from build123d import *

# Parameters (mm, degrees)
SKETCH1_W               = 120
SKETCH1_H               = 100
BOSS_EXTRUDE1_DEPTH     = 5
SKETCH2_R               = 2.5
CUT_EXTRUDE1_DEPTH      = 6
CUT_EXTRUDE3_DEPTH      = 10
BOSS_EXTRUDE3_DEPTH     = 60
SKETCH8_W               = 20
SKETCH8_H               = 5
BOSS_EXTRUDE4_DEPTH     = 65
SKETCH9_R               = 2.5
CUT_EXTRUDE4_DEPTH      = 71
BOSS_EXTRUDE5_DEPTH     = 5
SKETCH11_W              = 5
SKETCH11_H              = 70
CUT_EXTRUDE6_DEPTH      = 1
CUT_EXTRUDE6_DEPTH_BACK = 120.643960247
SKETCH12_R              = 1.5
CUT_EXTRUDE7_DEPTH      = 66
CUT_EXTRUDE7_DEPTH_BACK = 6
SKETCH13_W              = 69.121998964
SKETCH13_H              = 5
BOSS_EXTRUDE6_DEPTH     = 10
SKETCH14_R              = 1.5
CUT_EXTRUDE8_DEPTH      = 61
SKETCH15_W              = 5
SKETCH15_H              = 15
BOSS_EXTRUDE7_DEPTH     = 10
SKETCH17_R              = 1.5
CUT_EXTRUDE9_DEPTH      = 61


with BuildPart() as part:
    # Sketch1 → Boss-Extrude1 (new body)
    with BuildSketch(Plane.XY):
        with Locations((60, 50)):
            Rectangle(SKETCH1_W, SKETCH1_H)
    extrude(amount=BOSS_EXTRUDE1_DEPTH)

    # Sketch2 → Cut-Extrude1 (cut, through all)
    with BuildSketch(Plane.XY.offset(5)):
        with Locations((50.878001036, 56.909722104)):
            Circle(SKETCH2_R)
        with BuildLine():
            ThreePointArc((85.579375435, 7.351023424), (95.403755905, 15.949898455), (103.154556632, 26.456286582))
            ThreePointArc((103.154556632, 26.456286582), (98.465291161, 44.232978888), (80.688598855, 39.543713418))
            ThreePointArc((80.688598855, 39.543713418), (76.268720755, 33.552467296), (70.66638809, 28.648976576))
            ThreePointArc((70.66638809, 28.648976576), (67.473905187, 10.543506327), (85.579375435, 7.351023424))
        make_face()
    extrude(amount=-CUT_EXTRUDE1_DEPTH, mode=Mode.SUBTRACT)

    # Sketch5 → Cut-Extrude3 (cut)
    with BuildSketch(Plane.XY.offset(5)):
        with BuildLine():
            Line((120, 70), (50.878001036, 70))
            ThreePointArc((50.878001036, 70), (43.464411706, 67.698330385), (38.657892056, 61.602728806))
            Line((38.657892056, 61.602728806), (15, 0))
            Line((15, 0), (0, 0))
            Line((0, 0), (0, 100))
            Line((0, 100), (120, 100))
            Line((120, 100), (120, 70))
        make_face()
    extrude(amount=-CUT_EXTRUDE3_DEPTH, mode=Mode.SUBTRACT)

    # Sketch7 → Boss-Extrude3 (add)
    with BuildSketch(Plane(origin=(0, 0, 0), x_dir=(-1, 0, 0), z_dir=(0, 0, -1))):
        Polygon((-15, 0), (-37.603180225, 58.856367181), (-41.980029807, 56.306656226), (-20.356039753, 0), align=None)
        with BuildLine():
            Line((-120, 70), (-50.878001036, 70))
            ThreePointArc((-50.878001036, 70), (-49.44782984, 69.92163917), (-48.034781184, 69.687494847))
            Line((-48.034781184, 69.687494847), (-51.317000411, 65))
            Line((-51.317000411, 65), (-120, 65))
            Line((-120, 65), (-120, 70))
        make_face()
    extrude(amount=BOSS_EXTRUDE3_DEPTH)

    # Sketch8 → Boss-Extrude4 (add, through all)
    with BuildSketch(Plane(origin=(0, 0, -60), x_dir=(-1, 0, 0), z_dir=(0, 0, -1))):
        with Locations((-10.356039753, 2.5)):
            Rectangle(SKETCH8_W, SKETCH8_H)
    extrude(amount=-BOSS_EXTRUDE4_DEPTH)

    # Sketch9 → Cut-Extrude4 (cut, through all)
    with BuildSketch(Plane(origin=(0, 70, 0), x_dir=(1, 0, 0), z_dir=(0, 1, 0))):
        with Locations((108, 52)):
            Circle(SKETCH9_R)
    extrude(amount=-CUT_EXTRUDE4_DEPTH, mode=Mode.SUBTRACT)

    # Sketch10 → Boss-Extrude5 (add)
    with BuildSketch(Plane(origin=(0, 0, 0), x_dir=(-1, 0, 0), z_dir=(0, 0, -1))):
        with BuildLine():
            Line((-38.657892056, 61.602728806), (-37.603180225, 58.856367181))
            Line((-37.603180225, 58.856367181), (-41.980029807, 56.306656226))
            Line((-41.980029807, 56.306656226), (-43.482905887, 60.219991674))
            ThreePointArc((-43.482905887, 60.219991674), (-46.657937411, 63.826106989), (-51.317000411, 65))
            Line((-51.317000411, 65), (-48.034781184, 69.687494847))
            ThreePointArc((-48.034781184, 69.687494847), (-42.330087293, 66.823780104), (-38.657892056, 61.602728806))
        make_face()
    extrude(amount=BOSS_EXTRUDE5_DEPTH)

    # Sketch11 → Cut-Extrude6 (cut, two sides)
    with BuildSketch(Plane(origin=(120, 0, 0), x_dir=(0, 0, -1), z_dir=(1, 0, 0))) as cut_extrude6_sk:
        with Locations((-2.5, 35)):
            Rectangle(SKETCH11_W, SKETCH11_H)
    extrude(amount=CUT_EXTRUDE6_DEPTH, mode=Mode.SUBTRACT)
    extrude(cut_extrude6_sk.sketch, amount=-CUT_EXTRUDE6_DEPTH_BACK, mode=Mode.SUBTRACT)

    # Sketch12 → Cut-Extrude7 (cut, two sides)
    with BuildSketch(Plane(origin=(0, 5, 0), x_dir=(1, 0, 0), z_dir=(0, 1, 0))) as cut_extrude7_sk:
        with Locations((7.856039753, 10)):
            Circle(SKETCH12_R)
        with Locations((7.856039753, 50)):
            Circle(SKETCH12_R)
    extrude(amount=CUT_EXTRUDE7_DEPTH, mode=Mode.SUBTRACT)
    extrude(cut_extrude7_sk.sketch, amount=-CUT_EXTRUDE7_DEPTH_BACK, mode=Mode.SUBTRACT)

    # Sketch13 → Boss-Extrude6 (add)
    with BuildSketch(Plane(origin=(0, 70, 0), x_dir=(1, 0, 0), z_dir=(0, 1, 0))):
        with Locations((85.439000518, 2.5)):
            Rectangle(SKETCH13_W, SKETCH13_H)
        with Locations((85.439000518, 57.5)):
            Rectangle(SKETCH13_W, SKETCH13_H)
    extrude(amount=BOSS_EXTRUDE6_DEPTH)

    # Sketch14 → Cut-Extrude8 (cut, through all)
    with BuildSketch(Plane.XY):
        with Locations((65, 75)):
            Circle(SKETCH14_R)
        with Locations((115, 75)):
            Circle(SKETCH14_R)
    extrude(amount=-CUT_EXTRUDE8_DEPTH, mode=Mode.SUBTRACT)

    # Sketch15 → Boss-Extrude7 (add)
    with BuildSketch(Plane(origin=(13.072049518, -5.020185671, 0), x_dir=(0, 0, 1), z_dir=(-0.933525558, 0.358510854, 0))):
        with Locations((-2.5, 60.925071268)):
            Rectangle(SKETCH15_W, SKETCH15_H)
        with Locations((-57.5, 60.925071268)):
            Rectangle(SKETCH15_W, SKETCH15_H)
    extrude(amount=BOSS_EXTRUDE7_DEPTH)

    # Sketch17 → Cut-Extrude9 (cut, through all)
    with BuildSketch(Plane.XY):
        with Locations((30.246721032, 53.647479763)):
            Circle(SKETCH17_R)
    extrude(amount=-CUT_EXTRUDE9_DEPTH, mode=Mode.SUBTRACT)


solid = part.part
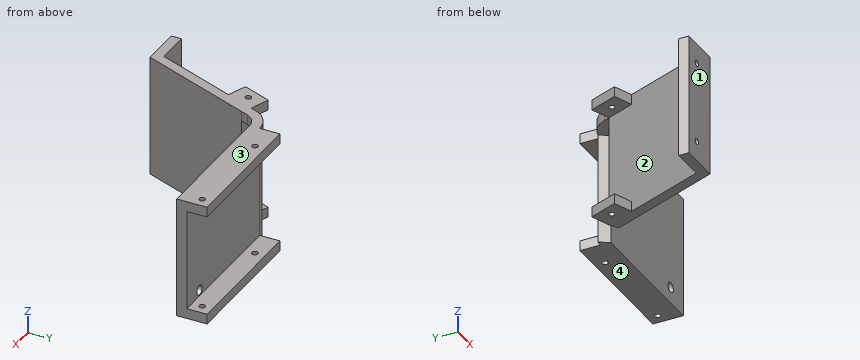
Verification items for the finished model (mm, model axes). Face numbers are marked on the shaded views. Round coordinates to 2 decimals unless told otherwise and drop trailing zeros. Loops run counter-clockwise (first coordinate to the right, second up) from the corner with the lowest first, then second, coordinate; pieces in that order, holes last. Notation, with made-up numbers: (81.5, 4) - (123.5, 4) arc R27 cw to (123.5, 32) - close; hole circle Ø11 at (84, 81.5). An arc over 180 degrees is marked (long way). Use one line per item in the form item = value.
1. Draft check along Z on the marked faces 1, 2, 3 and 4. Enter one of: pulls with the +Z half, pulls with the -Z half, needs draft (parallel to the pull), parting line crosses it, or undercut.
A:
face_1 = needs draft
face_2 = undercut
face_3 = pulls with the +Z half
face_4 = pulls with the -Z half
2. Section check D-D on x = 81. Record the cut outline in (y, z).
A:
outline = (65, -60) - (80, -60) - (80, -55) - (70, -55) - (70, -5) - (80, -5) - (80, 0) - (65, 0) - close
3. Section check A-A on z = -33.5. Record the cut outline in (x, y), and give its area (3 significant figures).
A:
outline = (0.36, 0) - (20.36, 0) - (41.98, 56.31) - (37.6, 58.86) - (16.92, 5) - (0.36, 5) - close; (48.03, 69.69) - (51.32, 65) - (120, 65) - (120, 70) - (50.88, 70) arc R13.09 ccw to start
area = 738 mm²
4. Scan lines: probe 1 along X at (y, z) = (75, -2); probe 2 along Y at (x, z) = (65, -2.5); probe 3 along X at (y, z) = (67.35, -52). Record each from-to range of solid material in increasing order.
A:
probe_1 = 50.88 to 63.5, 66.5 to 113.5, 116.5 to 120
probe_2 = 65 to 73.5, 76.5 to 80
probe_3 = 49.67 to 105.5, 110.5 to 120
5. Gauge pin test, flat ends, axial feed: pin 1 Ø1.5 at (y, z) = (73.5, -2) entering from -X; pin 2 Ø2.5 at (x, y) = (115, 75) entering from -Z; pin 3 Ø15 at (x, z) = (87, -27.5) entering from +Y; pin 4 Ø5 at (x, z) = (11, -24) entering from +Y. Record the tip position at first contact, or that the pin passes through.
A:
pin_1 = 50.88
pin_2 = through
pin_3 = 70
pin_4 = 5
6. Section check C-C on z = -10. Record the cut outline in (x, y), and give its area (3 significant figures).
A:
outline = (0.36, 0) - (6.36, 0) - (6.36, 5) - (0.36, 5) - close; (9.36, 0) - (20.36, 0) - (41.98, 56.31) - (37.6, 58.86) - (16.92, 5) - (9.36, 5) - close; (48.03, 69.69) - (51.32, 65) - (120, 65) - (120, 70) - (50.88, 70) arc R13.09 ccw to start
area = 723 mm²
7. Section check B-B on x = 108. Record the cut outline in (y, z), and give its area (3 significant figures).
A:
outline = (65, -60) - (80, -60) - (80, -55) - (70, -55) - (70, -54.5) - (65, -54.5) - close; (65, -49.5) - (70, -49.5) - (70, -5) - (80, -5) - (80, 0) - (65, 0) - close
area = 375 mm²
